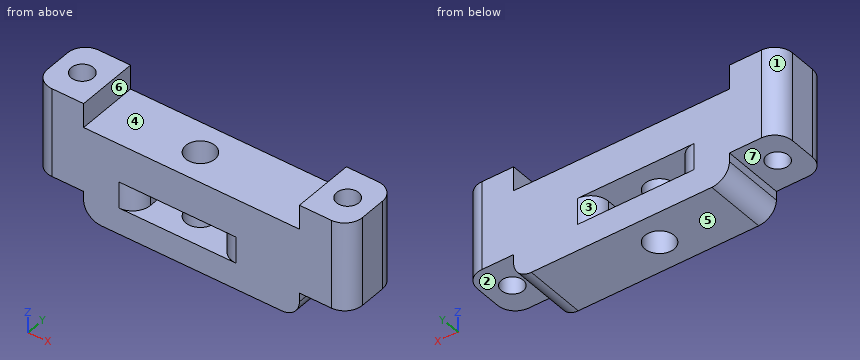
```python
from build123d import *

# Parameters (mm, degrees)
SKETCH1_W           = 9.175
SKETCH1_H           = 3
BOSS_EXTRUDE1_DEPTH = 3.5
SKETCH2_R           = 1.25
SKETCH2_R_2         = 1.65
CUT_EXTRUDE1_DEPTH  = 14.1
SKETCH3_W           = 5.6
SKETCH3_H           = 7
CUT_EXTRUDE2_DEPTH  = 3
FILLET1_R           = 2


with BuildPart() as part:
    # Sketch1 → Boss-Extrude1 (new body, symmetric)
    with BuildSketch(Plane(origin=(0, 0, 0), x_dir=(1, 0, 0), z_dir=(0, 1, 0))):
        Polygon((-17.8, 10.35), (17.8, 10.35), (17.8, -2.75), (12.2, -2.75), (12.2, 0), (-12.2, 0), (-12.2, -2.75), (-17.8, -2.75), align=None)
        with Locations((-1.5875, 5.85)):
            Rectangle(SKETCH1_W, SKETCH1_H, mode=Mode.SUBTRACT)
    extrude(amount=BOSS_EXTRUDE1_DEPTH, both=True)

    # Sketch2 → Cut-Extrude1 (cut, through all)
    with BuildSketch(Plane(origin=(0, 0, -10.35), x_dir=(-1, 0, 0), z_dir=(0, 0, -1))):
        with Locations((15, 0)):
            Circle(SKETCH2_R)
        with Locations((1.65, 0)):
            Circle(SKETCH2_R_2)
        with Locations((-15, 0)):
            Circle(SKETCH2_R)
    extrude(amount=-CUT_EXTRUDE1_DEPTH, mode=Mode.SUBTRACT)

    # Sketch3 → Cut-Extrude2 (cut)
    with BuildSketch(Plane(origin=(0, 0, -10.35), x_dir=(-1, 0, 0), z_dir=(0, 0, -1))):
        with Locations((15, 0)):
            Rectangle(SKETCH3_W, SKETCH3_H)
        with Locations((-15, 0)):
            Rectangle(SKETCH3_W, SKETCH3_H)
    extrude(amount=-CUT_EXTRUDE2_DEPTH, mode=Mode.SUBTRACT)

    # Fillet1
    fillet1_edges = [part.edges().sort_by_distance(p)[0] for p in [
        (17.8, -3.5, -2.3),
        (-6.175, -3.5, -5.85),
        (3, -3.5, -5.85),
        (-6.175, 3.5, -5.85),
        (3, 3.5, -5.85),
        (-17.8, -3.5, -2.3),
        (-17.8, 3.5, -2.3),
        (-12.2, 0, -10.35),
        (17.8, 3.5, -2.3),
        (12.2, 0, -10.35),
    ]]
    fillet(fillet1_edges, radius=FILLET1_R)


solid = part.part
```
The listing builds one solid part. Answer for the finished solid, in the listing's coordinates (mm). Face numbers are marked on the shaded views. A direction names the side the tool comes from. Round coordinates to 2 decimals unless told otherwise and drop trailing zeros. Loops run counter-clockwise (first coordinate to the right, second up) from the corner with the lowest first, then second, coordinate; pieces in that order, holes last.
Q1. Which of the six approach directions +Z, -Z, +X, -X, +Y, -Y give full straight-line access (tool end or side, diameter ignored) to the marked faces 5, 6 and 7?
Q2. For a pull along Z with two mould halves and no side action, classify the marked faces 1, 2, 3 and 4 as released by +Z, released by -Z, zero draft, split by the parting line, or undercut.
Q3. Section A-A, the plane x = -1.65 is taken. Determine the outline of the cut face in (y, z), then the cut area to 3 significant figures.
Q4. Section B-B, the plane x = -15 is taken. Determine the outline of the cut face in (y, z).
Q5. Section C-C, the plane y = 0 is taken. Count the separate pieces of the cut face and the enclosed holes in it, then the cut area to 3 significant figures.
Q6. Given pin 1 Ø1.5 at (x, y) = (-3, -2.5) entering from +Z; pin 2 Ø1.1 at (y, z) = (-1, -8) entering from -X; pin 3 Ø3 at (x, y) = (-14, 0.5) entering from -Z; pin 4 Ø0.8 at (y, z) = (1, -7.5) entering from +X, each flat-ended and moving along its own axis, determine where each tip first touches the part or whether it passes through.
Q7. Find the intervals of material crossed by line 1 (Y direction, x = -15, z = -3.5); line 2 (X direction, y = 0.25, z = -5.5) (3 decimals); line 3 (Z direction, x = -3, y = 3.25), in increasing order.
Q8. Section D-D, the plane z = -0.75 is taken. Determine the outline of the cut face in (x, y).
Completed:
1. face 5: -Z, +X, -X, +Y, -Y
1. face 6: +Z, +Y, -Y
1. face 7: -Z, -X, +Y, -Y
2. face 1: zero draft
2. face 2: released by -Z
2. face 3: undercut
2. face 4: released by +Z
3. outline: (-3.5, -10.35) - (-1.65, -10.35) - (-1.65, -7.35) - (-3.5, -7.35) - close; (-3.5, -4.35) - (-1.65, -4.35) - (-1.65, 0) - (-3.5, 0) - close; (1.65, -10.35) - (3.5, -10.35) - (3.5, -7.35) - (1.65, -7.35) - close; (1.65, -4.35) - (3.5, -4.35) - (3.5, 0) - (1.65, 0) - close
3. area: 27.2 mm2
4. outline: (-3.5, -7.35) - (-1.25, -7.35) - (-1.25, 2.75) - (-3.5, 2.75) - close; (1.25, -7.35) - (3.5, -7.35) - (3.5, 2.75) - (1.25, 2.75) - close
5. separate pieces: 4
5. enclosed holes: 0
5. area: 262 mm2
6. pin 1: stops at z = 0
6. pin 2: stops at x = -12.2
6. pin 3: stops at z = -7.35
6. pin 4: stops at x = 17.8
7. line 1: y = -3.5 to -1.25, 1.25 to 3.5
7. line 2: x = -17.8 to -16.225, -13.775 to -6.175, 3 to 13.775, 16.225 to 17.8
7. line 3: z = -10.35 to -7.35, -4.35 to 0
8. outline: (-17.8, -1.5) arc R2 ccw to (-15.8, -3.5) - (15.8, -3.5) arc R2 ccw to (17.8, -1.5) - (17.8, 1.5) arc R2 ccw to (15.8, 3.5) - (-15.8, 3.5) arc R2 ccw to (-17.8, 1.5) - close; hole circle Ø2.5 at (-15, 0); hole circle Ø3.3 at (-1.65, 0); hole circle Ø2.5 at (15, 0)
